Could you check a few things on this drawing? It's one solid part, dimensions in mm from its lowest x, y, z. A direction names the side the tool comes from. Round coordinates to 2 decimals unless told otherwise and drop trailing zeros. Write each loop counter-clockwise with the first axis right and the second up, starting at its lowest first coordinate (ties: lowest second). Pieces come first, ordered by that corner, then holes. Notation, with made-up numbers: (-6, -8) - (-1, -8) arc R17 cw to (-1, 17) - close; hole circle Ø5 at (-4.75, 37). An arc over 180 degrees is marked (long way). Put each result on its own line as item: value.
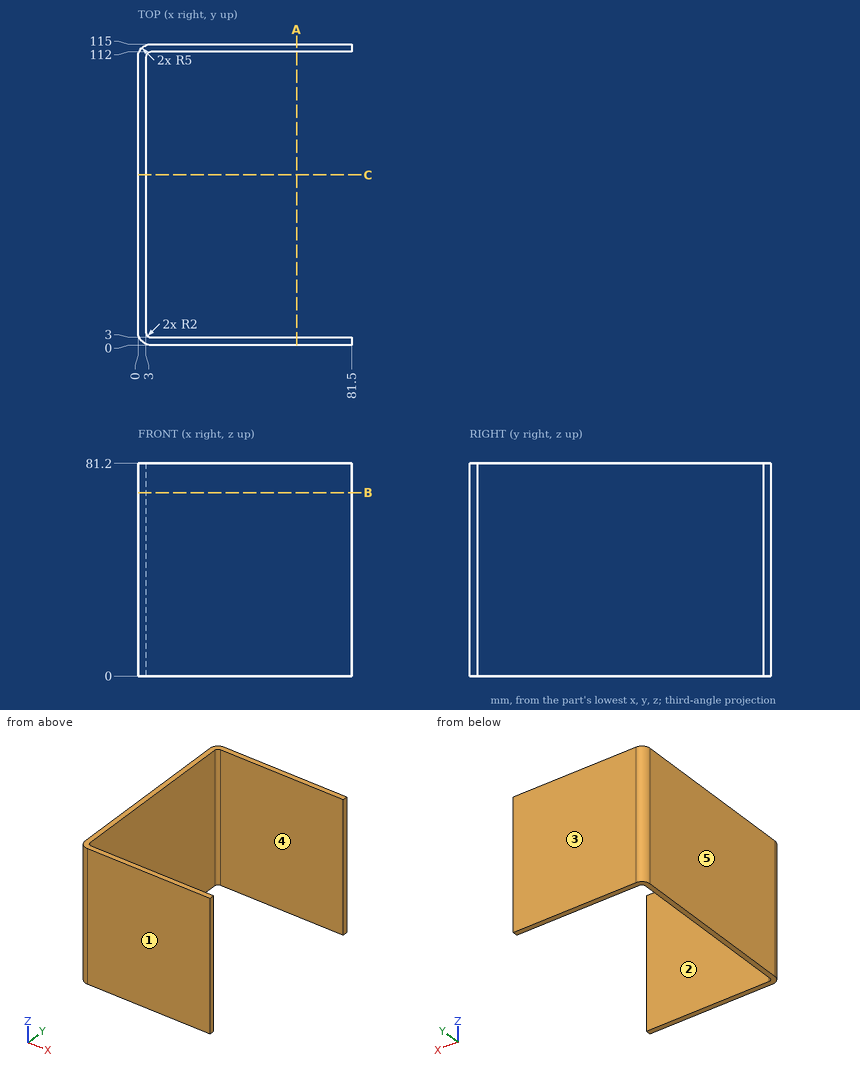
(1) For the marked faces 1 and 2, which set-ups out of +Z, -Z, +X, -X, +Y, -Y let a thin tool reach every point of the face, with its end or its side?
Values found:
face 1: +Z, -Z, +X, -X, -Y
face 2: +Z, -Z, +X
(2) Imagine slicing it at A-A, the plane x = 60.5. List the corners of the cut face in (y, z) for me, then the cut area to 3 significant figures.
Values found:
outline: (0, 0) - (3, 0) - (3, 81.2) - (0, 81.2) - close; (112, 0) - (115, 0) - (115, 81.2) - (112, 81.2) - close
area: 487 mm^2
(3) If we mould it in two halves opening along Y, with no side actions, what happens to the marked faces 3, 4 and 5? For each: pulls with the +Y half, pulls with the -Y half, needs draft (parallel to the pull), parting line crosses it, or undercut.
Values found:
face 3: pulls with the +Y half
face 4: undercut
face 5: needs draft
(4) Imagine slicing it at B-B, the plane z = 70. List the corners of the cut face in (x, y) for me.
Values found:
outline: (0, 5) arc R5 ccw to (5, 0) - (81.5, 0) - (81.5, 3) - (5, 3) arc R2 cw to (3, 5) - (3, 110) arc R2 cw to (5, 112) - (81.5, 112) - (81.5, 115) - (5, 115) arc R5 ccw to (0, 110) - close
(5) I'm going to push a flat-ended pin straight in: pin 1 (10 mm diameter, centred on y = 41.5, z = 11, fed in from +X). Where does the tip first touch, or does it pass through?
Values found:
pin 1: stops at x = 3
(6) Imagine slicing it at C-C, the plane y = 65. List the corners of the cut face in (x, z) for me.
Values found:
outline: (0, 0) - (3, 0) - (3, 81.2) - (0, 81.2) - close
(7) Please list where these lines run through material, in increasing order: probe 1 along Y at (x, z) = (72, 66); probe 2 along X at (y, z) = (45.5, 61.5). Write a range as from..to.
Values found:
probe 1: y = 0..3, 112..115
probe 2: x = 0..3
